Work out the finished part from the listing and answer in its coordinate system (mm). A direction names the side the tool comes from. Give positions to 0.01 mm unless a question says otherwise; leave off trailing zeros. Order: outer loops, then holes, each group sorted by start corner. A loop starts at its lowest first (then second) coordinate and runs counter-clockwise, first axis right, second up.
Autodesk Inventor part; units mm, degrees
ref_plane "YZ Plane" through (0, 0, 0) normal (1, 0, 0) x (0, 1, 0)
ref_plane "XZ Plane" through (0, 0, 0) normal (0, 1, 0) x (-1, 0, 0)
ref_plane "XY Plane" through (0, 0, 0) normal (0, 0, 1) x (1, 0, 0)
sketch "Sketch1" plane through (0, 0, 0) normal (0, 1, 0) x (-1, 0, 0)
  circle A0 centre (0, 0) radius 6.5
  circle A1 centre (0, 0) radius 10
  dimension "d0" = 13
  dimension "d1" = 20
extrude "Extrusion1" add sketch "Sketch1" along normal blind 30
sketch "Sketch2" plane through (0, 0, 0) normal (0, -1, 0) x (1, 0, 0)
  circle A0 centre (0, 0) radius 6
  circle A1 centre (0, 0) radius 6.5
  dimension "d4" = 12
extrude "Extrusion2" add sketch "Sketch2" against normal blind 15
sketch "Sketch3" plane through (0, 0, 0) normal (0, -1, 0) x (1, 0, 0)
  circle A0 centre (0, 0) radius 7.15
  dimension "d7" = 14.3
extrude "Extrusion3" cut sketch "Sketch3" against normal blind 5
fillet "Fillet1" radius 2 1 edges at (10, 30, 0)
sketch "Sketch4" plane through (0, 0, 0) normal (0, 0, 1) x (1, 0, 0)
  circle A0 centre (0, 12) radius 2.5
  line L0 (-8, 30) -> (8, 30)
  point P0 (0, 0)
  dimension "d11" = 5
  dimension "d12" = 18
extrude "Extrusion4" cut sketch "Sketch4" against normal blind 10
properties part number "ConnectorC"
1. Given P1, Ø7, axis at x = -0.5, z = 3, coming from the -Y side; P2, Ø10, axis at x = -4, z = 1, coming from the -Y side; P3, Ø1, axis at y = 7.5, z = -4.5, coming from the -X side; P4, Ø8, axis at x = 0, z = 0, coming from the -Y side, each flat-ended and moving along its own axis, determine where each tip first touches the part or whether it passes through.
Findings below:
P1: stops at y = 5
P2: stops at y = 0
P3: stops at x = -9.17
P4: passes through
2. The part is cut by section D-D (y = 12). Write down the section's boundary in (x, z).
Findings below:
outline: (-2.5, -9.68) - (-2.5, -5.45) arc R6 cw (long way) to (2.5, -5.45) - (2.5, -9.68) arc R10 ccw (long way) to start
3. The part is cut by section C-C (y = 3). Write down the section's boundary in (x, z), then the cut area to 3 significant figures.
Findings below:
outline: circle Ø20 at (0, 0); hole circle Ø14.3 at (0, 0)
area: 154 mm2
4. The mould has two halves that part along Z. Classify faces 1 (the face through (2.17, 13.8, 9.76)), 2 (the face through (-0.93, 2.46, 7.09)), 3 (the face through (-0.54, 9.56, -7.7)): pulls with the +Z half, pulls with the -Z half, needs draft (parallel to the pull), parting line crosses it, or undercut.
Findings below:
face 1: parting line crosses it
face 2: undercut
face 3: needs draft
5. Which of the six approach directions +Z, -Z, +X, -X, +Y, -Y give full straight-line access (tool end or side, diameter ignored) to faces 4 (the face through (5.158, 22.395, 3.955)), 5 (the face through (-2, 5, 6)), 6 (the face through (0, 30, 7))?
Findings below:
face 4: +Y
face 5: -Y
face 6: +Z, -Z, +X, -X, +Y
6. Straight lines are drawn through the part: probe 1 along Z at (x, y) = (0, 25.5); probe 2 along Z at (x, y) = (0, 1.2); probe 3 along X at (y, z) = (12, -7). For each, find the intervals that lie inside material, in ascending order.
Findings below:
probe 1: z = -10 to -6.5, 6.5 to 10
probe 2: z = -10 to -7.15, 7.15 to 10
probe 3: x = -7.14 to -2.5, 2.5 to 7.14
7. The part is cut by section B-B (x = 0). Write down the section's boundary in (y, z), then the cut area to 3 significant figures.
Findings below:
outline: (0, -10) - (9.5, -10) - (9.5, -6) - (5, -6) - (5, -7.15) - (0, -7.15) - close; (0, 7.15) - (5, 7.15) - (5, 6) - (15, 6) - (15, 6.5) - (30, 6.5) - (30, 8) arc R2 ccw to (28, 10) - (0, 10) - close; (14.5, -10) - (28, -10) arc R2 ccw to (30, -8) - (30, -6.5) - (15, -6.5) - (15, -6) - (14.5, -6) - close
area: 192 mm2
8. The part is cut by section A-A (z = 0). Write down the section's boundary in (x, y), then the cut area to 3 significant figures.
Findings below:
outline: (-10, 0) - (-7.15, 0) - (-7.15, 5) - (-6, 5) - (-6, 15) - (-6.5, 15) - (-6.5, 30) - (-8, 30) arc R2 ccw to (-10, 28) - close; (6, 5) - (7.15, 5) - (7.15, 0) - (10, 0) - (10, 28) arc R2 ccw to (8, 30) - (6.5, 30) - (6.5, 15) - (6, 15) - close
area: 212 mm2
